from build123d import *

# Parameters (mm, degrees)
F0_R     = 6.35
F1_DEPTH = 5.08
F2_R     = 6.35
F3_DEPTH = 38.1


# Not quite as in the source:
# - a feature names something its author has since deleted; it is built from what else it names


with BuildPart() as f1:
    # F0 (on Top) → F1 (new body)
    with BuildSketch(Plane.XY):
        with BuildLine():
            ThreePointArc((-164.7597998381, -122.2357259512), (-149.8808243223, -158.1567504355), (-113.9597998381, -173.0357259512))
            Line((-113.9597998381, -173.0357259512), (117.6952974319, -173.0357259512))
            ThreePointArc((117.6952974319, -173.0357259512), (153.6163219162, -158.1567504355), (168.4952974319, -122.2357259512))
            Line((168.4952974319, -122.2357259512), (168.4952974319, 114.9484769821))
            ThreePointArc((168.4952974319, 114.9484769821), (153.6163219162, 150.8695014664), (117.6952974319, 165.7484769821))
            Line((117.6952974319, 165.7484769821), (-113.9597998381, 165.7484769821))
            ThreePointArc((-113.9597998381, 165.7484769821), (-149.8808243223, 150.8695014664), (-164.7597998381, 114.9484769821))
            Line((-164.7597998381, 114.9484769821), (-164.7597998381, -122.2357259512))
        make_face()
        with BuildLine():
            ThreePointArc((-69.85, -21.7389110476), (-33.9289755157, -36.6178865633), (-19.05, -72.5389110476))
            Line((-19.05, -72.5389110476), (-19.05, -107.3567504355))
            ThreePointArc((-19.05, -107.3567504355), (-33.9289755157, -143.2777749197), (-69.85, -158.1567504355))
            Line((-69.85, -158.1567504355), (-99.0808243223, -158.1567504355))
            ThreePointArc((-99.0808243223, -158.1567504355), (-135.0018488066, -143.2777749197), (-149.8808243223, -107.3567504355))
            Line((-149.8808243223, -107.3567504355), (-149.8808243223, -72.5389110476))
            ThreePointArc((-149.8808243223, -72.5389110476), (-135.0018488066, -36.6178865633), (-99.0808243223, -21.7389110476))
            Line((-99.0808243223, -21.7389110476), (-69.85, -21.7389110476))
        make_face(mode=Mode.SUBTRACT)
        Polygon((-19.05, -158.1567504355), (0, -107.3567504355), (19.05, -158.1567504355), align=None, mode=Mode.SUBTRACT)
        with BuildLine():
            Line((69.85, -21.7389110476), (102.8163219162, -21.7389110476))
            ThreePointArc((102.8163219162, -21.7389110476), (138.7373464005, -36.6178865633), (153.6163219162, -72.5389110476))
            Line((153.6163219162, -72.5389110476), (153.6163219162, -107.3567504355))
            ThreePointArc((153.6163219162, -107.3567504355), (138.7373464005, -143.2777749197), (102.8163219162, -158.1567504355))
            Line((102.8163219162, -158.1567504355), (69.85, -158.1567504355))
            ThreePointArc((69.85, -158.1567504355), (33.9289755157, -143.2777749197), (19.05, -107.3567504355))
            Line((19.05, -107.3567504355), (19.05, -72.5389110476))
            ThreePointArc((19.05, -72.5389110476), (33.9289755157, -36.6178865633), (69.85, -21.7389110476))
        make_face(mode=Mode.SUBTRACT)
        Polygon((-149.8808243223, -21.7389110476), (-149.8808243223, 16.3610889524), (-99.0808243223, 0), align=None, mode=Mode.SUBTRACT)
        Circle(F0_R, mode=Mode.SUBTRACT)
        with BuildLine():
            ThreePointArc((-69.85, 150.8695014664), (-33.9289755157, 135.9905259507), (-19.05, 100.0695014664))
            Line((-19.05, 100.0695014664), (-19.05, 67.1610889524))
            ThreePointArc((-19.05, 67.1610889524), (-33.9289755157, 31.2400644681), (-69.85, 16.3610889524))
            Line((-69.85, 16.3610889524), (-99.0808243223, 16.3610889524))
            ThreePointArc((-99.0808243223, 16.3610889524), (-135.0018488066, 31.2400644681), (-149.8808243223, 67.1610889524))
            Line((-149.8808243223, 67.1610889524), (-149.8808243223, 100.0695014664))
            ThreePointArc((-149.8808243223, 100.0695014664), (-135.0018488066, 135.9905259507), (-99.0808243223, 150.8695014664))
            Line((-99.0808243223, 150.8695014664), (-69.85, 150.8695014664))
        make_face(mode=Mode.SUBTRACT)
        Polygon((19.05, 150.8695014664), (0, 100.0695014664), (-19.05, 150.8695014664), align=None, mode=Mode.SUBTRACT)
        Polygon((153.6163219162, -21.7389110476), (102.8163219162, 0), (153.6163219162, 16.3610889524), align=None, mode=Mode.SUBTRACT)
        with BuildLine():
            ThreePointArc((153.6163219162, 67.1610889524), (138.7373464005, 31.2400644681), (102.8163219162, 16.3610889524))
            Line((102.8163219162, 16.3610889524), (69.85, 16.3610889524))
            ThreePointArc((69.85, 16.3610889524), (33.9289755157, 31.2400644681), (19.05, 67.1610889524))
            Line((19.05, 67.1610889524), (19.05, 100.0695014664))
            ThreePointArc((19.05, 100.0695014664), (33.9289755157, 135.9905259507), (69.85, 150.8695014664))
            Line((69.85, 150.8695014664), (102.8163219162, 150.8695014664))
            ThreePointArc((102.8163219162, 150.8695014664), (138.7373464005, 135.9905259507), (153.6163219162, 100.0695014664))
            Line((153.6163219162, 100.0695014664), (153.6163219162, 67.1610889524))
        make_face(mode=Mode.SUBTRACT)
    extrude(amount=F1_DEPTH)

    # F2 (on Top) → F3 (join)
    with BuildSketch(Plane.XY):
        with Locations((-142.0295983553, -152.4900346994)):
            Circle(F2_R)
        with Locations((-142.0295983553, 144.2388147116)):
            Circle(F2_R)
        with Locations((147.0908075571, 144.2388147116)):
            Circle(F2_R)
        with Locations((147.0908075571, -152.4900346994)):
            Circle(F2_R)
    extrude(amount=-F3_DEPTH)


solid = f1.part
Design review of the part built by this model. Coordinates are the model's own, in mm. A direction names the side the tool comes from. Give positions to 0.01 mm unless a question says otherwise; leave off trailing zeros. Write each loop counter-clockwise with the first axis right and the second up, starting at its lowest first coordinate (ties: lowest second). Pieces come first, ordered by that corner, then holes. Notation, with made-up numbers: M -25,58 L 19,58 A23 ccw 19,94 Z; hole C 80,-38 d9. An arc over 180 degrees is marked long. Answer as a JSON object with one key per item and string values. Group by question number.
1) We need section A-A (x = 91.5). Give the boundary of the cut face in (y, z), and give its area (3 significant figures).
2) We need section C-C (z = -8). Give the boundary of the cut face in (x, y), and give its area (3 significant figures).
3) For line 1 along Z through (x, y) = (-140, 31); line 2 along Y through (x, z) = (-26.5, 3); line 3 along X through (y, z) = (139, -1.5), list the stretches that pass through material, from the lowest coordinate up.
4) Mouldability with a two-part tool opening along Y and no side actions: class faces 1 (the face through (139.13, 31.637, 2.504)), 2 (the face through (-142, 144, -38.1)), 3 (the face through (-150.274, -157.76, 2.504)) as released by +Y, released by -Y, zero draft, split by the parting line, or undercut.
5) Tool access review of faces 4 (the face through (150.505, 149.593, -18.783)), 5 (the face through (138.34, 136.383, 2.504)), 6 (the face through (147, -152, -38.1)): name each direction out of +Z, -Z, +X, -X, +Y, -Y from which nothing blocks a thin tool from reaching the whole face with its end or side.
6) We need section B-B (y = 57.5). Give the boundary of the cut face in (x, z).
7) Clearance check with flat-ended pins moving along their axes: pin 1 Ø6 at (x, z) = (131, -1.5) entering from -Y; pin 2 Ø1 at (x, y) = (2, 3.5) entering from +Z; pin 3 Ø10 at (x, y) = (-69.5, -2) entering from -Z. State where each tip first meets the part, or that it passes through.
Answer key:
{
 "1": {"outline": "M -173.04,0 L -158.16,0 L -158.16,5.08 L -173.04,5.08 Z; M -21.74,0 L 16.36,0 L 16.36,5.08 L -21.74,5.08 Z; M 150.87,0 L 165.75,0 L 165.75,5.08 L 150.87,5.08 Z", "area": "345 mm²"},
 "2": {"outline": "C -142.03,-152.49 d12.7; C -142.03,144.24 d12.7; C 147.09,-152.49 d12.7; C 147.09,144.24 d12.7", "area": "507 mm²"},
 "3": {"line 1": "z = 0 to 5.08", "line 2": "y = -173.04 to -133.84, -46.05 to 40.68, 126.55 to 165.75", "line 3": "x = -145.62 to -138.44, 143.5 to 150.68"},
 "4": {"face 1": "undercut", "face 2": "zero draft", "face 3": "released by -Y"},
 "5": {"face 4": "-Z", "face 5": "+Z, -Z", "face 6": "-Z, +X, -X, +Y, -Y"},
 "6": {"outline": "M -164.76,0 L -148.95,0 L -148.95,5.08 L -164.76,5.08 Z; M -19.98,0 L 19.98,0 L 19.98,5.08 L -19.98,5.08 Z; M 152.69,0 L 168.5,0 L 168.5,5.08 L 152.69,5.08 Z"},
 "7": {"pin 1": "stops at y = -171.89", "pin 2": "passes through", "pin 3": "stops at z = 0"}
}
